Read the model definition and answer for the solid it produces. Units are mm, in the model's axes. A direction names the side the tool comes from. Round coordinates to 2 decimals unless told otherwise and drop trailing zeros. Loops run counter-clockwise (first coordinate to the right, second up) from the corner with the lowest first, then second, coordinate; pieces in that order, holes last. Notation, with made-up numbers: M -26,-35.5 L -11,-35.5 A31 cw -11,3.5 Z; hole C -21,16.25 d8. An arc over 180 degrees is marked long. Answer as CSV lines item,"result".
```python
from build123d import *

# Parameters (mm, degrees)
SKETCH1_R           = 4.5
SKETCH1_R_2         = 3.25
BOSS_EXTRUDE1_DEPTH = 20
SKETCH2_W           = 20
SKETCH2_H           = 10
BOSS_EXTRUDE2_DEPTH = 1.25
FILLET1_R           = 2
SKETCH3_R           = 2
BOSS_EXTRUDE3_DEPTH = 12
LPATTERN3_COUNT     = 2
LPATTERN3_PITCH     = 14.5
FILLET2_R           = 1


with BuildPart() as part:
    # Sketch1 → Boss-Extrude1 (new body)
    with BuildSketch(Plane(origin=(0, 0, 0), x_dir=(1, 0, 0), z_dir=(0, 1, 0))):
        with Locations(Location((0, 0, 0), (0, 0, 270))):
            Circle(SKETCH1_R)
        with Locations(Location((0, 0, 0), (0, 0, 270))):
            Circle(SKETCH1_R_2, mode=Mode.SUBTRACT)
    extrude(amount=BOSS_EXTRUDE1_DEPTH)

    # Sketch2 → Boss-Extrude2 (add, symmetric)
    with BuildSketch(Plane.XY.offset(-4.5)):
        with Locations((0, 15)):
            Rectangle(SKETCH2_W, SKETCH2_H)
    extrude(amount=BOSS_EXTRUDE2_DEPTH, both=True)

    # Fillet1
    fillet1_edges = [part.edges().sort_by_distance(p)[0] for p in [
        (-10, 10, -4.5),
        (10, 10, -4.5),
        (10, 20, -4.5),
        (-10, 20, -4.5),
    ]]
    fillet(fillet1_edges, radius=FILLET1_R)

    # Sketch3 → Boss-Extrude3 (add)
    with BuildSketch(Plane(origin=(0, 0, -5.75), x_dir=(-1, 0, 0), z_dir=(0, 0, -1))):
        with Locations((-7.25, 15)):
            Circle(SKETCH3_R)
    boss_extrude3 = extrude(amount=BOSS_EXTRUDE3_DEPTH)

    # LPattern3: Boss-Extrude3 ×2
    with Locations(*[(-i * LPATTERN3_PITCH, 0, 0) for i in range(1, LPATTERN3_COUNT)]):
        add(boss_extrude3)

    # Fillet2
    fillet2_edges = [part.edges().sort_by_distance(p)[0] for p in [
        (9.25, 15, -17.75),
        (-5.25, 15, -17.75),
    ]]
    fillet(fillet2_edges, radius=FILLET2_R)


solid = part.part
```
1) A tool of negligible diameter and unlimited length cuts with its end or side. For faces 1 (the flat face through (-7, 15, -3.25)), 2 (the flat face through (7, 15, -3.25)), 3 (the cylindrical face through (8.724, 16.352, -11.173)), from which of +Z, -Z, +X, -X, +Y, -Y can it reach the whole face along a straight path? Write none if from no direction.
Evaluation:
face 1,"-X, +Y, -Y"
face 2,"+X, +Y, -Y"
face 3,"-Z"
2) Find section A-A, the plane z = 0. Give the vertices of the cut face in (x, y).
Evaluation:
outline,"M -4.5,0 L -3.25,0 L -3.25,20 L -4.5,20 Z; M 3.25,0 L 4.5,0 L 4.5,20 L 3.25,20 Z"
3) Find section C-C, the plane y = 6.25. Give the vertices of the cut face in (x, z).
Evaluation:
outline,"C 0,0 d9; hole C 0,0 d6.5"
4) Determine the mould class of faces 4 (the cylindrical face through (-1.978, 9.86, -2.579)), 5 (the cylindrical face through (-5.776, 16.352, -11.173)), 6 (the flat face through (7, 15, -17.75)) for opening direction Z: released by +Z, released by -Z, zero draft, split by the parting line, or undercut.
Evaluation:
face 4,"undercut"
face 5,"zero draft"
face 6,"released by -Z"
5) Find section D-D, the plane z = -7. Give the vertices of the cut face in (x, y).
Evaluation:
outline,"C -7.25,15 d4; C 7.25,15 d4"
6) Each of these flat-tipped pins is pushed along its axis until it touches: P1, Ø2, axis at x = -7.5, y = 15, coming from the +Z side; P2, Ø4, axis at y = 16.5, z = -0.5, coming from the -X side; P3, Ø2, axis at x = 6, z = 0, coming from the -Y side; P4, Ø8, axis at x = 7.5, y = 15, coming from the +Z side. Where does it stop, or does it pass through?
Evaluation:
P1,"stops at z = -3.25"
P2,"stops at x = -4.5"
P3,"passes through"
P4,"stops at z = 2.83"
7) Find section B-B, the plane x = -3.75. Give the vertices of the cut face in (y, z).
Evaluation:
outline,"M 0,-2.49 L 20,-2.49 L 20,2.49 L 0,2.49 Z; M 10,-5.75 L 20,-5.75 L 20,-3.25 L 10,-3.25 Z"
8) Straight lines are drawn through the part: line 1 (X direction, y = 10.5, z = 0); line 2 (Z direction, x = 0, y = 15). For each, find the intervals that lie inside material, in ascending order.
Evaluation:
line 1,"x = -4.5 to -3.25, 3.25 to 4.5"
line 2,"z = -5.75 to -3.25, 3.25 to 4.5"
